from build123d import *

# Parameters (mm, degrees)
SKETCH2_R           = 20.5
BOSS_EXTRUDE1_DEPTH = 20
SKETCH3_R           = 2.5
CUT_EXTRUDE1_DEPTH  = 20
CIRPATTERN1_COUNT   = 6


with BuildPart() as part:
    # Sketch2 → Boss-Extrude1 (new body)
    with BuildSketch(Plane(origin=(0, 0, 0), x_dir=(1, 0, 0), z_dir=(0, 1, 0))):
        with BuildLine():
            Line((22.113344387, 80), (-22.113344387, 80))
            ThreePointArc((-22.113344387, 80), (-41.5, 71.880108514), (-58.225360109, 59.150718002))
            Line((-58.225360109, 59.150718002), (-80.338704497, 20.849281998))
            ThreePointArc((-80.338704497, 20.849281998), (-83, 0), (-80.338704497, -20.849281998))
            Line((-80.338704497, -20.849281998), (-58.225360109, -59.150718002))
            ThreePointArc((-58.225360109, -59.150718002), (-41.5, -71.880108514), (-22.113344387, -80))
            Line((-22.113344387, -80), (22.113344387, -80))
            ThreePointArc((22.113344387, -80), (41.5, -71.880108514), (58.225360109, -59.150718002))
            Line((58.225360109, -59.150718002), (80.338704497, -20.849281998))
            ThreePointArc((80.338704497, -20.849281998), (83, 0), (80.338704497, 20.849281998))
            Line((80.338704497, 20.849281998), (58.225360109, 59.150718002))
            ThreePointArc((58.225360109, 59.150718002), (41.5, 71.880108514), (22.113344387, 80))
        make_face()
        with Locations(Location((0, 0, 0), (0, 0, 270))):
            Circle(SKETCH2_R, mode=Mode.SUBTRACT)
        with BuildLine():
            Line((-15.519237886, 66.880108514), (15.519237886, 66.880108514))
            ThreePointArc((15.519237886, 66.880108514), (24.179491924, 61.880108514), (24.179491924, 51.880108514))
            Line((24.179491924, 51.880108514), (17.320508076, 40))
            ThreePointArc((17.320508076, 40), (0, 30), (-17.320508076, 40))
            Line((-17.320508076, 40), (-24.179491924, 51.880108514))
            ThreePointArc((-24.179491924, 51.880108514), (-24.179491924, 61.880108514), (-15.519237886, 66.880108514))
        make_face(mode=Mode.SUBTRACT)
        with BuildLine():
            Line((50.160254038, 46.880108514), (65.679491924, 20))
            ThreePointArc((65.679491924, 20), (65.679491924, 10), (57.019237886, 5))
            Line((57.019237886, 5), (43.301270189, 5))
            ThreePointArc((43.301270189, 5), (25.980762114, 15), (25.980762114, 35))
            Line((25.980762114, 35), (32.839745962, 46.880108514))
            ThreePointArc((32.839745962, 46.880108514), (41.5, 51.880108514), (50.160254038, 46.880108514))
        make_face(mode=Mode.SUBTRACT)
        with BuildLine():
            Line((65.679491924, -20), (50.160254038, -46.880108514))
            ThreePointArc((50.160254038, -46.880108514), (41.5, -51.880108514), (32.839745962, -46.880108514))
            Line((32.839745962, -46.880108514), (25.980762114, -35))
            ThreePointArc((25.980762114, -35), (25.980762114, -15), (43.301270189, -5))
            Line((43.301270189, -5), (57.019237886, -5))
            ThreePointArc((57.019237886, -5), (65.679491924, -10), (65.679491924, -20))
        make_face(mode=Mode.SUBTRACT)
        with BuildLine():
            Line((15.519237886, -66.880108514), (-15.519237886, -66.880108514))
            ThreePointArc((-15.519237886, -66.880108514), (-24.179491924, -61.880108514), (-24.179491924, -51.880108514))
            Line((-24.179491924, -51.880108514), (-17.320508076, -40))
            ThreePointArc((-17.320508076, -40), (0, -30), (17.320508076, -40))
            Line((17.320508076, -40), (24.179491924, -51.880108514))
            ThreePointArc((24.179491924, -51.880108514), (24.179491924, -61.880108514), (15.519237886, -66.880108514))
        make_face(mode=Mode.SUBTRACT)
        with BuildLine():
            Line((-50.160254038, -46.880108514), (-65.679491924, -20))
            ThreePointArc((-65.679491924, -20), (-65.679491924, -10), (-57.019237886, -5))
            Line((-57.019237886, -5), (-43.301270189, -5))
            ThreePointArc((-43.301270189, -5), (-25.980762114, -15), (-25.980762114, -35))
            Line((-25.980762114, -35), (-32.839745962, -46.880108514))
            ThreePointArc((-32.839745962, -46.880108514), (-41.5, -51.880108514), (-50.160254038, -46.880108514))
        make_face(mode=Mode.SUBTRACT)
        with BuildLine():
            Line((-65.679491924, 20), (-50.160254038, 46.880108514))
            ThreePointArc((-50.160254038, 46.880108514), (-41.5, 51.880108514), (-32.839745962, 46.880108514))
            Line((-32.839745962, 46.880108514), (-25.980762114, 35))
            ThreePointArc((-25.980762114, 35), (-25.980762114, 15), (-43.301270189, 5))
            Line((-43.301270189, 5), (-57.019237886, 5))
            ThreePointArc((-57.019237886, 5), (-65.679491924, 10), (-65.679491924, 20))
        make_face(mode=Mode.SUBTRACT)
    extrude(amount=BOSS_EXTRUDE1_DEPTH)

    # Sketch3 → Cut-Extrude1 (cut)
    with BuildSketch(Plane.XY.offset(80)):
        with Locations((0, 10)):
            Circle(SKETCH3_R)
    cut_extrude1 = extrude(amount=-CUT_EXTRUDE1_DEPTH, mode=Mode.SUBTRACT)

    # CirPattern1: Cut-Extrude1 ×6 about axis
    cirpattern1_axis = Axis((0, 20, 0), (0, 1, 0))
    for i in range(1, CIRPATTERN1_COUNT):
        add(cut_extrude1.rotate(cirpattern1_axis, i * 360 / CIRPATTERN1_COUNT), mode=Mode.SUBTRACT)


solid = part.part
Geometry check sheet. Reference: the model listing, model coordinates, mm. A direction names the side the tool comes from. Round coordinates to 2 decimals unless told otherwise and drop trailing zeros. Loops run counter-clockwise (first coordinate to the right, second up) from the corner with the lowest first, then second, coordinate; pieces in that order, holes last. Notation, with made-up numbers: (25.25, 25) - (60.25, 25) arc R15 ccw to (60.25, 44) - close; hole circle Ø3 at (73.25, 20). An arc over 180 degrees is marked (long way). One line per question, with ' | ' between items. Start each with the question number.
1. Cross-section at A-A on z = 0. Record the cut outline in (x, y), then the cut area to 3 significant figures.
2. Depth check by flat-ended pin: pin 1 (7 mm diameter, centred on x = -50, y = 5.5, fed in from -Z); pin 2 (6 mm diameter, centred on y = 12.5, z = -26.5, fed in from +X); pin 3 (1 mm diameter, centred on x = -42.5, z = 6.5, fed in from +Y); pin 4 (7 mm diameter, centred on x = -50, y = 9.5, fed in from +Z). Enter the tip coordinate at first touch or a pass-through.
3. Draft check along X on faces 3 (the face through (-29.458, 9.86, -41.023)), 4 (the face through (0, 5, -80)), 5 (the face through (69.44, 5.42, -39.73)). Enter one of: released by +X, released by -X, zero draft, split by the parting line, or undercut.
4. Tool access check on faces 1 (the face through (29.458, 9.86, 41.023)), 2 (the face through (0, 5, 80)). Record the directions out of +Z, -Z, +X, -X, +Y, -Y that give a thin tool (end or side, any length) a straight path to the whole face; none if there is none.
5. Cross-section at B-B on x = 0. Record the cut outline in (y, z).
6. Cross-section at C-C on y = 5. State how many separate pieces and enclosed holes the cut face has, then the cut area to 3 significant figures.
7. Scan lines: line 1 (Z direction, x = -64, y = 18.5); line 2 (Y direction, x = 0, z = 72); line 3 (Z direction, x = -36, y = 17.25). Record each from-to range of solid material in increasing order. Write a range as [from, to].
Taken from the geometry:
1) outline: (-83, 0) - (-20.5, 0) - (-20.5, 20) - (-83, 20) - close; (20.5, 0) - (83, 0) - (83, 20) - (20.5, 20) - close | area: 2,500 mm²
2) pin 1: z = -68.75 | pin 2: x = 78.81 | pin 3: through | pin 4: z = 68.75
3) face 3: undercut | face 4: zero draft | face 5: released by +X
4) face 1: +Y, -Y | face 2: +Z, +X, -X, +Y, -Y
5) outline: (0, -80) - (7.5, -80) - (7.5, -66.88) - (0, -66.88) - close; (0, -30) - (20, -30) - (20, -20.5) - (0, -20.5) - close; (0, 20.5) - (20, 20.5) - (20, 30) - (0, 30) - close; (0, 66.88) - (7.5, 66.88) - (7.5, 80) - (0, 80) - close; (12.5, -80) - (20, -80) - (20, -66.88) - (12.5, -66.88) - close; (12.5, 66.88) - (20, 66.88) - (20, 80) - (12.5, 80) - close
6) separate pieces: 1 | enclosed holes: 7 | area: 11,000 mm²
7) line 1: [-49.15, -22.91], [-7.84, 7.84], [22.91, 49.15] | line 2: [0, 7.5], [12.5, 20] | line 3: [-74.79, -50.23], [-6.38, 6.38], [50.23, 74.79]
